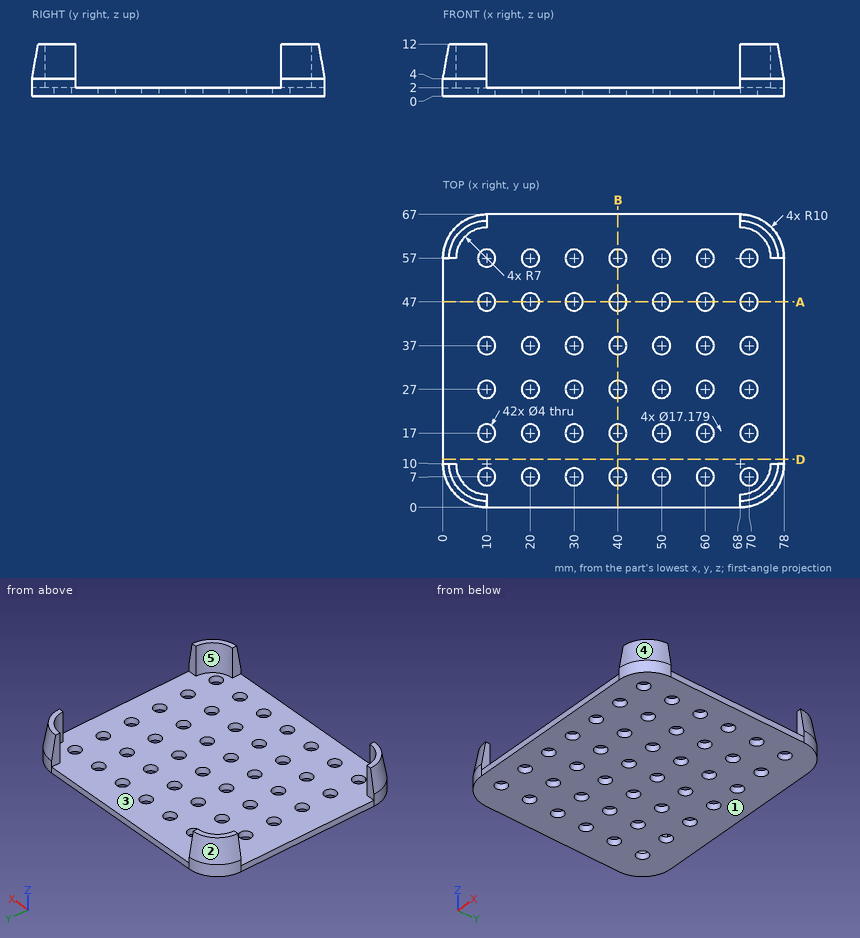
Verification items for this drawing (mm, ordinates from the low corner). A direction names the side the tool comes from. Round coordinates to 2 decimals unless told otherwise and drop trailing zeros. Order: outer loops, then holes, each group sorted by start corner. A loop starts at its lowest first (then second) coordinate and runs counter-clockwise, first axis right, second up.
1) Cross-section at A-A, the plane y = 47. Give the number of separate pieces and of enclosed holes in the cut face, plus the area to 3 significant figures.
Geometry says:
separate pieces: 8
enclosed holes: 0
area: 100 mm2
2) Tool access check on the marked faces 4 and 5. Record the directions out of +Z, -Z, +X, -X, +Y, -Y that give a thin tool (end or side, any length) a straight path to the whole face; none if there is none.
Geometry says:
face 4: +Z, +X, -Y
face 5: +Z
3) Material ranges on line 1 (Y direction, x = 68.5, z = 4); line 2 (Z direction, x = 33, y = 49); line 3 (X direction, y = 5, z = 5) (1 decimal), recorded low to high.
Geometry says:
line 1: y = 0.01 to 3.02, 63.98 to 66.99
line 2: z = 0 to 2
line 3: x = 1.5 to 5.1, 72.9 to 76.5
4) Draft check along X on the marked faces 1, 2 and 3. Enter one of: +X half, -X half, draft (parallel to the pull), parting line (faces both ways), or undercut.
Geometry says:
face 1: draft
face 2: -X half
face 3: undercut
5) Depth check by flat-ended pin: pin 1 (3.5 mm diameter, centred on x = 50, y = 17, fed in from -Z); pin 2 (2.5 mm diameter, centred on x = 2, z = 6.5, fed in from +Y); pin 3 (20 mm diameter, centred on x = 24.5, y = 31, fed in from +Z); pin 4 (1.5 mm diameter, centred on y = 66, z = 7.5, fed in from +X). Enter the tip coordinate at first touch or a pass-through.
Geometry says:
pin 1: passes through
pin 2: stops at y = 63.81
pin 3: stops at z = 2
pin 4: stops at x = 72.5
6) Cross-section at B-B, the plane x = 40. Record the cut outline in (y, z).
Geometry says:
outline: (0, 0) - (5, 0) - (5, 2) - (0, 2) - close; (9, 0) - (15, 0) - (15, 2) - (9, 2) - close; (19, 0) - (25, 0) - (25, 2) - (19, 2) - close; (29, 0) - (35, 0) - (35, 2) - (29, 2) - close; (39, 0) - (45, 0) - (45, 2) - (39, 2) - close; (49, 0) - (55, 0) - (55, 2) - (49, 2) - close; (59, 0) - (67, 0) - (67, 2) - (59, 2) - close
7) Cross-section at D-D, the plane y = 11. Record the cut outline in (x, z).
Geometry says:
outline: (0, 0) - (78, 0) - (78, 2) - (0, 2) - close
